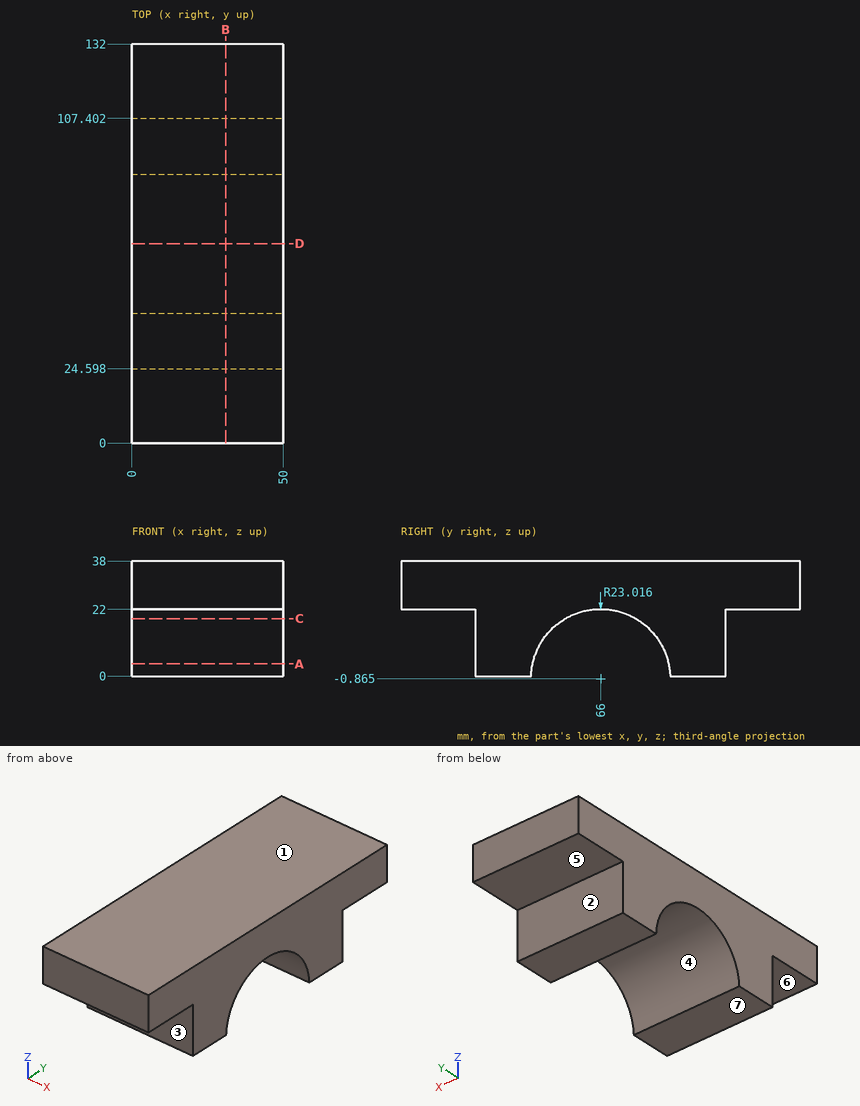
Part print with two shaded views. Sizes in mm from the minimum x, y, z corner. A direction names the side the tool comes from. Coordinates: 2 decimals unless noted, no trailing zeros. Write each loop counter-clockwise with the first axis right and the second up, starting at its lowest first coordinate (ties: lowest second). Pieces come first, ordered by that corner, then holes. Notation, with made-up numbers: (70, 10) - (111, 10) arc R35 cw to (111, 48) - close; hole circle Ø10 at (67.5, -36.5). An arc over 180 degrees is marked (long way). Use a Markdown table: item, result. Add a question column.
Item 1: Band-saw the part on B-B, the plane x = 31. Write the cut outline in (y, z) (1 decimal).
Item 2: Drop flat-ended pins along their axis: pin 1 (12 mm diameter, centred on y = 41, z = 32.5, fed in from -X); pin 2 (1.5 mm diameter, centred on x = 44.5, z = 12.5, fed in from -Y); pin 3 (8 mm diameter, centred on x = 31, y = 79, fed in from -Z); pin 4 (12.5 mm diameter, centred on x = 36.5, y = 114, fed in from -Z). Give the stop position or say it passes through.
Item 3: 3-axis set-ups, long thin cutter, end or side, ignore diameter. For the marked faces 5, 6 and 7: which of +Z, -Z, +X, -X, +Y, -Y reach the whole face in a straight line?
Item 4: Band-saw the part on C-C, the plane z = 19. Write the cut outline in (x, y).
Item 5: Band-saw the part on D-D, the plane y = 66. Write the cut outline in (x, z).
Item 6: Two-plate mould, pull along Y, no slides. Class the marked faces 1, 2, 3 and 4: pulls with the +Y half, pulls with the -Y half, needs draft (parallel to the pull), parting line crosses it, or undercut.
Item 7: Band-saw the part on A-A, the plane z = 4. Write the cut outline in (x, y), and give its area (3 significant figures).
Item 8: Drill centre lines: line 1 along Y through (x, z) = (42.5, 16); line 2 along Y through (x, z) = (14.5, 14); line 3 along Z through (x, y) = (5, 112.5). Where is each one in solid material? Low to high.
A:
| question | item | result |
|---|---|---|
| 1 | outline | (0, 22) - (24.6, 22) - (24.6, 0) - (43, 0) arc R23 cw to (89, 0) - (107.4, 0) - (107.4, 22) - (132, 22) - (132, 38) - (0, 38) - close |
| 2 | pin 1 | stops at x = 0 |
| 2 | pin 2 | stops at y = 24.6 |
| 2 | pin 3 | stops at z = 14.65 |
| 2 | pin 4 | stops at z = 22 |
| 3 | face 5 | -Z, +X, -X, +Y |
| 3 | face 6 | -Z, +X, -X, -Y |
| 3 | face 7 | -Z, +X, -X, +Y, -Y |
| 4 | outline | (0, 24.6) - (50, 24.6) - (50, 54.38) - (0, 54.38) - close; (0, 77.62) - (50, 77.62) - (50, 107.4) - (0, 107.4) - close |
| 5 | outline | (0, 22.15) - (50, 22.15) - (50, 38) - (0, 38) - close |
| 6 | face 1 | needs draft |
| 6 | face 2 | pulls with the +Y half |
| 6 | face 3 | pulls with the -Y half |
| 6 | face 4 | undercut |
| 7 | outline | (0, 24.6) - (50, 24.6) - (50, 43.5) - (0, 43.5) - close; (0, 88.5) - (50, 88.5) - (50, 107.4) - (0, 107.4) - close |
| 7 | area | 1,890 mm² |
| 8 | line 1 | y = 24.6 to 50.34, 81.66 to 107.4 |
| 8 | line 2 | y = 24.6 to 48.43, 83.57 to 107.4 |
| 8 | line 3 | z = 22 to 38 |
